```python
from build123d import *

# Parameters (mm, degrees)
BOX_W     = 40
BOX_H     = 40
BOX_DEPTH = 3
FILLET_R  = 3


with BuildPart() as con001:
    # Cone001 → Cone001 (revolve)
    with BuildSketch(Plane(origin=(0, 0, -9), x_dir=(1, 0, 0), z_dir=(0, -1, 0))):
        Polygon((0, 0), (15, 0), (3, 50), (0, 50), align=None)
    revolve(axis=Axis((0, 0, -9), (0, 0, 1)))


with BuildPart() as fillet_body:
    # Box → Box (new body)
    with BuildSketch(Plane(origin=(-20, -20, 0), x_dir=(1, 0, 0), z_dir=(0, 0, 1))):
        with Locations((20, 20)):
            Rectangle(BOX_W, BOX_H)
    extrude(amount=BOX_DEPTH)

    # Fillet
    fillet_edges = [fillet_body.edges().sort_by_distance(p)[0] for p in [
        (-20, -20, 1.5),
        (-20, 20, 1.5),
        (20, -20, 1.5),
        (20, 20, 1.5),
    ]]
    fillet(fillet_edges, radius=FILLET_R)


with BuildPart() as cut:
    # Cone → Cone (revolve)
    with BuildSketch(Plane.XZ):
        Polygon((0, 0), (16, 0), (4, 40), (0, 40), align=None)
    revolve(axis=Axis((0, 0, 0), (0, 0, 1)))

    # Fusion: union Fillet body
    add(fillet_body.part)

    # Cut: cut Con001
    add(con001.part, mode=Mode.SUBTRACT)


with BuildPart() as cut_1:
    # Cut placement: moved
    add(cut.part.moved(Location((20, 20, 0))))


solid = cut_1.part
```
Check sheet for the modelled part. Datum: model origin and axes. Units: mm. Round coordinates to 2 decimals unless told otherwise and drop trailing zeros. Order: outer loops, then holes, each group sorted by start corner. A loop starts at its lowest first (then second) coordinate and runs counter-clockwise, first axis right, second up.
1) Section check A-A (x = 20). Record the boundary of the cut face in (y, z), and give its area (4 significant figures).
2) Section check D-D (y = 4). Record the boundary of the cut face in (x, z).
3) Mould release check, pull along X, two halves, no side actions. Record for faces 1 (the conical face through (13.67, 15.15, 20.28)), 2 (the flat face through (0, 20, 1)), 3 (the flat face through (11, 34, 3)): +X half, -X half, draft (parallel to the pull), parting line (faces both ways), or undercut.
4) Go/stop test with flat-tipped pins: pin 1 Ø8 at (y, z) = (32.5, 23) entering from -X; pin 2 Ø10 at (y, z) = (21, 19.5) entering from -X; pin 3 Ø3 at (x, z) = (18, 24) entering from -Y; pin 4 Ø6 at (y, z) = (7, 29) entering from -X. Record where each tip stops, or that it passes through.
5) Section check C-C (z = 23.5). Record the boundary of the cut face in (x, y), and give its area (3 significant figures).
6) Scan lines: line 1 (Z direction, x = 2, y = 3.5); line 2 (Y direction, x = 28, z = 2); line 3 (X direction, y = 14.5, z = 28.5). Record each from-to range of solid material in increasing order.
Result:
1. outline: (0, 0) - (7.16, 0) - (16.76, 40) - (16, 40) - (4.9, 3) - (0, 3) - close; (23.24, 40) - (32.84, 0) - (40, 0) - (40, 3) - (35.1, 3) - (24, 40) - close
1. area: 183.5 mm2
2. outline: (0, 0) - (40, 0) - (40, 3) - (0, 3) - close
3. face 1: undercut
3. face 2: -X half
3. face 3: draft
4. pin 1: stops at x = 16.25
4. pin 2: stops at x = 8.37
4. pin 3: stops at y = 10.89
4. pin 4: passes through
5. outline: circle Ø17.9 at (20, 20); hole circle Ø14.4 at (20, 20)
5. area: 88.8 mm2
6. line 1: z = 0 to 3
6. line 2: y = 0 to 10.58, 29.42 to 40
6. line 3: x = 14.97 to 17.6, 22.4 to 25.03
